Model file for the job. Use its own axes, mm. Face numbers are marked on the shaded views. A direction names the side the tool comes from. Give positions to 0.01 mm unless a question says otherwise; leave off trailing zeros. Order: outer loops, then holes, each group sorted by start corner. A loop starts at its lowest first (then second) coordinate and runs counter-clockwise, first axis right, second up. Notation, with made-up numbers: (0, -33.5) - (7, -33.5) arc R22 cw to (7, -18.5) - close; hole circle Ø4 at (22, 35.5). An arc over 180 degrees is marked (long way). Use CSV: the item, a comma, the result in double quotes. Start each with the question number.
(1) Band-saw the part on A-A, the plane z = 102. Give the cut face in (x, y).
(2) Tool access for the marked faces 1 and 2: list every direction of +Z, -Z, +X, -X, +Y, -Y with a clear straight run to the whole face (end or side of a thin tool).
(3) Band-saw the part on B-B, the plane z = 0. Give the cut face in (x, y).
(4) Pull direction X, two halves, no side cores. Call the marked faces 3, 4, 5 and 6: +X half, -X half, draft (parallel to the pull), parting line (faces both ways), or undercut.
(5) Probe L1, parallel to Z at x = 0, y = 74; L2, parallel to X at y = 124, z = 0; L3, parallel to X at y = 843.5, z = -119. List the from-to ranges inside material, lowest first.
(6) Drop flat-ended pins along their axis: pin 1 Ø6 at (x, y) = (-334, 291.5) entering from +Z; pin 2 Ø1.5 at (y, z) = (150, -187) entering from -X; pin 3 Ø4 at (x, z) = (-115.5, -11) entering from -Y. Give the stop position or say it passes through.
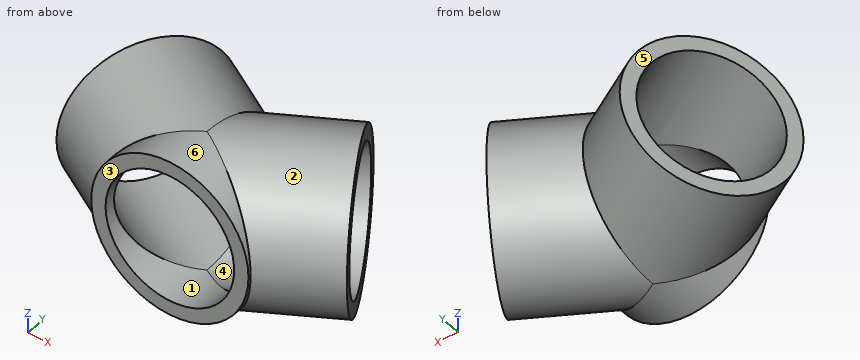
Autodesk Inventor part; units mm, degrees
ref_plane "Work Plane1" through (615.9173, 635, 0) normal (0.8660254, 0.5, 0) x (-0.5, 0.8660254, 0)
ref_plane "Work Plane2" through (-615.9173, 635, 0) normal (-0.8660254, 0.5, 0) x (-0.5, -0.8660254, 0)
ref_plane "YZ Plane" through (0, 0, 0) normal (1, 0, 0) x (0, 1, 0)
sketch "Sketch1" plane through (0, 0, 0) normal (0, 0, 1) x (1, 0, 0)
  line L0 (0, 0) -> (0, 279.4)
  line L1 (0, 279.4) -> (615.9173, 635)
  line L2 (0, 279.4) -> (-615.9173, 635)
  line L3 (-615.9173, 635) -> (615.9173, 635) construction
  dimension "A_dimension" = 279.4
  dimension "angle" = 120
  dimension "B_dimension" = 711.2
sketch "Sketch2" plane through (0, 0, 0) normal (0, 1, 0) x (-1, 0, 0)
  circle A0 centre (0, 0) radius 457.2
  circle A1 centre (0, 0) radius 373.9896
  dimension "outerDiameter" = 914.4
  dimension "wallThickness" = 83.2104
ref_plane "Work Plane1" through (615.9173, 635, 0) normal (0.8660254, 0.5, 0) x (-0.5, 0.8660254, 0)
sketch "Sketch3" plane through (615.9173, 635, 0) normal (0.8660254, 0.5, 0) x (-0.5, 0.8660254, 0)
  circle A0 centre (0, 0) radius 457.2
  circle A1 centre (0, 0) radius 373.9896
  point P0 (-241.9675, 0)
  point P1 (0, 0)
  dimension "d7" = 914.4
  dimension "d8" = 83.2104
ref_plane "Work Plane2" through (-615.9173, 635, 0) normal (-0.8660254, 0.5, 0) x (-0.5, -0.8660254, 0)
sketch "Sketch4" plane through (-615.9173, 635, 0) normal (-0.8660254, 0.5, 0) x (-0.5, -0.8660254, 0)
  circle A0 centre (0, 0) radius 457.2
  circle A1 centre (0, 0) radius 373.9896
  point P0 (241.9675, 0)
  point P1 (0, 0)
  dimension "d9" = 914.4
  dimension "d11" = 83.2104
extrude "Extrusion1" add sketch "Sketch2" along normal up to surface (279.4 mm away)
extrude "Extrusion2" add sketch "Sketch4" against normal up to surface (711.2 mm away)
extrude "Extrusion3" add sketch "Sketch3" against normal up to surface (711.2 mm away)
extrude "Extrusion4" cut sketch "Sketch2" along normal up to surface (279.4 mm away) contours A1
extrude "Extrusion5" cut sketch "Sketch3" against normal up to surface (711.2 mm away) contours A1
extrude "Extrusion6" cut sketch "Sketch4" against normal up to surface (711.2 mm away) contours A1
extrude "Extrusion7" cut sketch "Sketch4" along normal through all contours A0 | A1
extrude "Extrusion8" cut sketch "Sketch3" along normal through all contours A0 | A1
extrude "Extrusion9" cut sketch "Sketch2" against normal through all contours A0 | A1
equation "\"d7\" = outerDiameter"
equation "\"d8\" = wallThickness"
equation "\"d9\" = outerDiameter"
equation "\"d11\" = wallThickness"
equation "\"nominalSize\" = 914.4"
properties part number "WYE-S36-SCH160-120"
Answer block:
1,outline,"(-838.76, 249.03) - (-445.68, 22.09) - (-445.68, 0) - (-359.81, 0) - (-359.81, 71.66) - (-795.82, 323.39) - close; (-436.01, 946.61) - (0, 694.87) - (436.01, 946.61) - (393.08, 1020.97) - (0, 794.02) - (-393.08, 1020.97) - close; (359.81, 0) - (445.68, 0) - (445.68, 22.09) - (838.76, 249.03) - (795.82, 323.39) - (359.81, 71.66) - close"
2,face 1,"-Y"
2,face 2,"none"
3,outline,"(-844.52, 239.05) - (-457.2, 15.44) - (-457.2, 0) - (-373.99, 0) - (-373.99, 63.48) - (-802.91, 311.12) - close; (-428.92, 958.88) - (0, 711.25) - (428.92, 958.88) - (387.32, 1030.95) - (0, 807.33) - (-387.32, 1030.95) - close; (373.99, 0) - (457.2, 0) - (457.2, 15.44) - (844.52, 239.05) - (802.91, 311.12) - (373.99, 63.48) - close"
4,face 3,"draft"
4,face 4,"undercut"
4,face 5,"-X half"
4,face 6,"parting line"
5,L1,"z = -457.2 to -373.99, 373.99 to 457.2"
5,L2,"x = -645.24 to -478.82, 478.82 to 645.24"
5,L3,"x = -267.95 to -94.17, 94.17 to 267.95"
6,pin 1,"stops at z = 430.65"
6,pin 2,"stops at x = -611.75"
6,pin 3,"stops at y = 776.59"
